Solid Edge part; units mm, degrees
sketch "Sketch1" plane through (0, 0, 0) normal (0, 0, 1) x (1, 0, 0)
  line L0 (-15, -15) -> (15, -15)
  line L1 (15, -15) -> (15, 15)
  line L2 (15, 15) -> (-15, 15)
  line L3 (-15, 15) -> (-15, -15)
  dimension "D1" = 15
  dimension "D2" = 15
extrude "Protrusion1" add sketch "Sketch1" along normal blind 7
sketch "Sketch2" plane through (0, 0, 7) normal (0, 0, 1) x (0, 1, 0)
  circle A0 centre (11, 11) radius 1.5
  dimension "D1" = 11
extrude "Antenna" add sketch "Sketch2" along normal blind 20
fillet "Rotondo_1" radius 2 4 edges at (-15, 15, 3.5) (-15, -15, 3.5) (15, 15, 3.5) (15, -15, 3.5)
fillet "Rotondo_2" radius 2 1 edges at (-11, 9.5, 7)
chamfer "Smusso_1" distance 1 angle 45 1 edges at (-11, 9.5, 27)
sketch "Sketch3" plane through (0, 0, 7) normal (0, 0, 1) x (0, 1, 0)
  line L0 (8, -7.5) -> (8, -12.5)
  line L1 (8, -12.5) -> (13, -12.5)
  line L2 (13, -12.5) -> (13, -7.5)
  line L3 (13, -7.5) -> (8, -7.5)
extrude "Alloggio_Motori_1" add sketch "Sketch3" along normal blind 10
sketch "Sketch4" plane through (10, 13, 9) normal (0, 1, 0) x (-1, 0, 0)
  circle A0 centre (0, 0.5) radius 1
extrude "ScavoEstrusione_3" cut sketch "Sketch4" against normal blind 4
sketch "Sketch5" plane through (0, 0, 7) normal (0, 0, 1) x (0, 1, 0)
  line L0 (-12.5, 7.5) -> (-7.5, 7.5)
  line L1 (-7.5, 7.5) -> (-7.5, 12.5)
  line L2 (-7.5, 12.5) -> (-12.5, 12.5)
  line L3 (-12.5, 12.5) -> (-12.5, 7.5)
  dimension "D1" = 12.5
extrude "Alloggio_Motori_3" add sketch "Sketch5" along normal blind 10
sketch "Sketch6" plane through (12.5, 10.5, 12) normal (1, 0, 0) x (0, 1, 0)
  circle A0 centre (0, 2.5) radius 1
extrude "ScavoEstrusione_9" cut sketch "Sketch6" against normal blind 4
sketch "Sketch7" plane through (-12.5, -10, 12) normal (-1, 0, 0) x (0, -1, 0)
  circle A0 centre (0, -2.5) radius 1
extrude "ScavoEstrusione_10" cut sketch "Sketch7" against normal blind 4
sketch "Sketch8" plane through (-10, -12.5, 12) normal (0, -1, 0) x (1, 0, 0)
  circle A0 centre (0, 2.5) radius 1
extrude "ScavoEstrusione_11" cut sketch "Sketch8" against normal blind 4
sketch "Sketch9" plane through (0, 0, 7) normal (0, 0, 1) x (1, 0, 0)
  line L0 (7.5, -12.5) -> (12.5, -12.5)
  line L1 (12.5, -12.5) -> (12.5, -5.5)
  line L2 (12.5, -5.5) -> (7.5, -5.5)
  line L3 (7.5, -5.5) -> (7.5, -12.5)
  dimension "D1" = 7.5
  dimension "D2" = 12.5
extrude "Alloggio_collegamento" add sketch "Sketch9" along normal blind 10
sketch "Sketch10" plane through (12.5, -9, 12) normal (1, 0, 0) x (0, 1, 0)
  line L0 (-2.5, -1.5) -> (2.5, -1.5)
  line L1 (2.5, -1.5) -> (2.5, 1.5)
  line L2 (2.5, 1.5) -> (-2.5, 1.5)
  line L3 (-2.5, 1.5) -> (-2.5, -1.5)
  dimension "D1" = 2.5
  dimension "D2" = 2.5
extrude "ScavoEstrusione_12" cut sketch "Sketch10" against normal blind 4
Check sheet for the modelled part. Datum: model origin and axes. Units: mm. A direction names the side the tool comes from. Coordinates: 2 decimals unless noted, no trailing zeros. Loops run counter-clockwise (first coordinate to the right, second up) from the corner with the lowest first, then second, coordinate; pieces in that order, holes last. Notation, with made-up numbers: (78, 79) -> (126, 79) arc R27 cw to (126, 116) -> close; hole circle Ø6 at (2, -23). An arc over 180 degrees is marked (long way). Write item = value, one per line. Start each with the question number.
1. Section check A-A on z = 9.5. Record the cut outline in (x, y).
2. Tool access check on faces 1 (the flat face through (-10, -8.5, 15)), 2 (the cylindrical face through (10.528, 10.283, 13.524)), 3 (the cylindrical face through (-10.53, -9.87, 10.49)). Record the directions out of +Z, -Z, +X, -X, +Y, -Y that give a thin tool (end or side, any length) a straight path to the whole face; none if there is none.
3. Section check D-D on y = -4. Record the cut outline in (x, z), then the cut area to 3 significant figures.
4. Section check C-C on x = 10. Record the cut outline in (y, z), then the cut area to 3 significant figures.
5. Draft check along Y on faces 4 (the flat face through (-12.5, -10, 12)), 5 (the flat face through (8.5, -9, 12)), 6 (the flat face through (10, 8, 12)), 7 (the cylindrical face through (14.4, -14.43, 3.55)). Enter one of: released by +Y, released by -Y, zero draft, split by the parting line, or undercut.
6. Section check B-B on y = -10. Record the cut outline in (x, z), then the cut area to 3 significant figures.
7. Material ranges on line 1 (Z direction, x = -10.15, y = -10); line 2 (Z direction, x = -14, y = 13); line 3 (X direction, y = 10.75, z = 11.5), recorded low to high.
8. Depth check by flat-ended pin: P1, Ø3.5, axis at y = -8, z = 13, coming from the +X side; P2, Ø1.5, axis at x = 10.5, z = 14, coming from the -Y side; P3, Ø1.5, axis at x = 10.5, z = 14, coming from the +Y side. Enter the tip coordinate at first touch or a pass-through.
Responses:
q1.outline = (-12.5, -12.5) -> (-7.5, -12.5) -> (-7.5, -7.5) -> (-12.5, -7.5) -> (-12.5, -9) -> (-8.5, -9) -> (-8.5, -11) -> (-12.5, -11) -> close; circle Ø3 at (-11, 11); (7.5, -12.5) -> (12.5, -12.5) -> (12.5, -5.5) -> (7.5, -5.5) -> close; (7.5, 8) -> (12.5, 8) -> (12.5, 13) -> (11, 13) -> (11, 9) -> (9, 9) -> (9, 13) -> (7.5, 13) -> close
q2.face_1 = -Y
q2.face_2 = +X
q2.face_3 = -X
q3.outline = (-15, 0) -> (15, 0) -> (15, 7) -> (-15, 7) -> close
q3.area = 210 mm2
q4.outline = (-15, 0) -> (15, 0) -> (15, 7) -> (13, 7) -> (13, 8.5) -> (9, 8.5) -> (9, 10.5) -> (13, 10.5) -> (13, 17) -> (8, 17) -> (8, 7) -> (-5.5, 7) -> (-5.5, 17) -> (-12.5, 17) -> (-12.5, 7) -> (-15, 7) -> close; hole (-11.5, 10.5) -> (-6.5, 10.5) -> (-6.5, 13.5) -> (-11.5, 13.5) -> close; hole circle Ø2 at (10.5, 14.5)
q4.area = 304 mm2
q5.face_4 = zero draft
q5.face_5 = undercut
q5.face_6 = undercut
q5.face_7 = released by -Y
q6.outline = (-15, 0) -> (15, 0) -> (15, 7) -> (12.5, 7) -> (12.5, 10.5) -> (8.5, 10.5) -> (8.5, 13.5) -> (12.5, 13.5) -> (12.5, 17) -> (7.5, 17) -> (7.5, 7) -> (-7.5, 7) -> (-7.5, 17) -> (-12.5, 17) -> (-12.5, 10.5) -> (-8.5, 10.5) -> (-8.5, 8.5) -> (-12.5, 8.5) -> (-12.5, 7) -> (-15, 7) -> close; hole circle Ø2 at (-10, 14.5)
q6.area = 287 mm2
q7.line_1 = 0 to 8.5, 10.5 to 13.51, 15.49 to 17
q7.line_2 = 0 to 7
q7.line_3 = -12.48 to -9.52, 7.5 to 12.5
q8.P1 = 12.5
q8.P2 = -12.5
q8.P3 = 13
